Can you work these out from the model? Positions are in its coordinate system, mm. Face numbers are marked on the shaded views. A direction names the side the tool comes from. Give positions to 0.01 mm unless a question says otherwise; leave off trailing zeros. Order: outer loops, then holes, each group sorted by start corner. A loop starts at its lowest first (then second) coordinate and runs counter-clockwise, first axis right, second up.
```python
from build123d import *
from build123d.topology import SkipClean

# Parameters (mm, degrees)
BOSS_EXTRUDE1_START = -12.5
SKETCH1_W           = 27
SKETCH1_H           = 33
SKETCH1_R           = 7
BOSS_EXTRUDE1_DEPTH = 17
BOSS_EXTRUDE3_DEPTH = 12.5
BOSS_EXTRUDE4_START = 12.5
SKETCH1_5_R         = 5
BOSS_EXTRUDE4_DEPTH = 7
CHAMFER1_SIZE       = 5


with BuildPart() as part:
    # Sketch1 → Boss-Extrude1 (new body)
    with BuildSketch(Plane.XY.offset(BOSS_EXTRUDE1_START)):
        with Locations((-33.967633793, -25.34)):
            Rectangle(SKETCH1_W, SKETCH1_H)
        with Locations((-31.467633793, -22.84)):
            Circle(SKETCH1_R, mode=Mode.SUBTRACT)
    extrude(amount=BOSS_EXTRUDE1_DEPTH)

    # Sketch1<4> → Boss-Extrude3 (add, symmetric)
    with BuildSketch(Plane.XY):
        with BuildLine():
            ThreePointArc((28.205719919, -40.677666444), (11.699513519, -31.708687123), (1.506567213, -15.928912557))
            ThreePointArc((1.506567213, -15.928912557), (-3.134727468, -15.689916625), (-7.511545005, -14.127161486))
            Line((-7.511545005, -14.127161486), (-17.455249537, -8.84))
            Line((-17.455249537, -8.84), (-20.467633793, -8.84))
            Line((-20.467633793, -8.84), (-20.467633793, -41.84))
            Line((-20.467633793, -41.84), (-18.535800645, -41.84))
            ThreePointArc((-18.535800645, -41.84), (-12.817002571, -43.63662578), (-9.153112508, -48.38093028))
            ThreePointArc((-9.153112508, -48.38093028), (-5.868981967, -55.429445297), (-1.467633793, -61.84))
            Line((-1.467633793, -61.84), (11.532366207, -61.84))
            Line((11.532366207, -61.84), (28.205719919, -40.677666444))
        make_face()
    extrude(amount=BOSS_EXTRUDE3_DEPTH, both=True)

    # Sketch1<5> → Boss-Extrude4 (add)
    with BuildSketch(Plane.XY.offset(BOSS_EXTRUDE4_START)):
        with BuildLine():
            Line((37.532366207, -3.84), (15.532366207, -3.84))
            ThreePointArc((15.532366207, -3.84), (10.445897028, -12.1195394), (1.506567213, -15.928912557))
            ThreePointArc((1.506567213, -15.928912557), (11.699513519, -31.708687123), (28.205719919, -40.677666444))
            Line((28.205719919, -40.677666444), (37.532366207, -28.84))
            Line((37.532366207, -28.84), (37.532366207, -3.84))
        make_face()
        with Locations((25.532366207, -18.84)):
            Circle(SKETCH1_5_R, mode=Mode.SUBTRACT)
    boss_extrude4 = extrude(amount=-BOSS_EXTRUDE4_DEPTH)

    # Mirror1: Boss-Extrude4 across plane
    with SkipClean():  # the faces are left unmerged after this step: merging them gives an invalid solid
        add(boss_extrude4.mirror(Plane.XY))

    # Chamfer1
    chamfer1_edges = [part.edges().sort_by_distance(p)[0] for p in [
        (-47.467633793, -41.84, -4),
        (-47.467633793, -8.84, -4),
        (37.532366207, -3.84, 9),
        (37.532366207, -3.84, -9),
    ]]
    chamfer(chamfer1_edges, length=CHAMFER1_SIZE)


solid = part.part
```
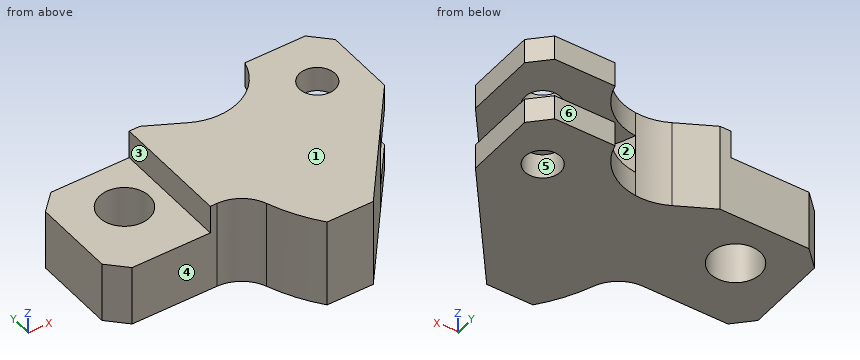
1) We'd pull the mould along Y, two halves only. Please class the marked faces 4, 5 and 6: +Y half, -Y half, draft (parallel to the pull), parting line (faces both ways), or undercut.
2) If I drill on line 1 (Z direction, x = 15.5, y = -30); line 2 (Y direction, x = -23.5, z = -8.25); line 3 (Y direction, x = 22, z = -6), over which ranges is the centre line in solid material (lowest first)?
3) I'm going to push flat-ended pins straight in: pin 1 Ø2.5 at (y, z) = (-23.5, 6.5) entering from -X; pin 2 Ø6 at (y, z) = (-35.5, 3) entering from +X; pin 3 Ø12 at (x, z) = (21.5, 1) entering from -Y. Where does each tip first touch, or does it pass through?
4) Suppose I cut it at B-B (z = 0). Please give me the cut outline in (x, y).
5) Suppose I cut it at C-C (y = -18.84). Please give me the cut outline in (x, z).
6) Suppose I cut it at A-A (z = -11). Please give me the cut outline in (x, y).
7) Suppose I cut it at D-D (x = 12.5). Please give me the cut outline in (y, z), and give its area (3 significant figures).
8) Which directions (+Z, -Z, +X, -X, +Y, -Y) give clear straight access to the entire face, cutting with the end or side of a thin tool? Please do the marked faces 1, 2 and 3.
Results:
1. face 4: -Y half
1. face 5: undercut
1. face 6: +Y half
2. line 1: z = -12.5 to -5.5, 5.5 to 12.5
2. line 2: y = -41.84 to -8.84
2. line 3: y = -48.55 to -22.38, -15.3 to -3.84
3. pin 1: stops at x = -20.47
3. pin 2: stops at x = 33.59
3. pin 3: stops at y = -56.8
4. outline: (-47.47, -36.84) - (-42.47, -41.84) - (-18.54, -41.84) arc R10 cw to (-9.15, -48.38) arc R47 ccw to (-1.47, -61.84) - (11.53, -61.84) - (28.21, -40.68) arc R38 cw to (1.51, -15.93) arc R16 cw to (-7.51, -14.13) - (-17.46, -8.84) - (-42.47, -8.84) - (-47.47, -13.84) - close; hole circle Ø14 at (-31.47, -22.84)
5. outline: (-47.47, -12.5) - (-37.21, -12.5) - (-37.21, 4.5) - (-47.47, 4.5) - close; (-25.72, -12.5) - (20.53, -12.5) - (20.53, -5.5) - (2.62, -5.5) - (2.62, 5.5) - (20.53, 5.5) - (20.53, 12.5) - (-20.47, 12.5) - (-20.47, 4.5) - (-25.72, 4.5) - close; (30.53, -12.5) - (37.53, -12.5) - (37.53, -5.5) - (30.53, -5.5) - close; (30.53, 5.5) - (37.53, 5.5) - (37.53, 12.5) - (30.53, 12.5) - close
6. outline: (-47.47, -36.84) - (-42.47, -41.84) - (-18.54, -41.84) arc R10 cw to (-9.15, -48.38) arc R47 ccw to (-1.47, -61.84) - (11.53, -61.84) - (37.53, -28.84) - (37.53, -8.84) - (32.53, -3.84) - (15.53, -3.84) arc R16 cw to (-7.51, -14.13) - (-17.46, -8.84) - (-42.47, -8.84) - (-47.47, -13.84) - close; hole circle Ø14 at (-31.47, -22.84); hole circle Ø10 at (25.53, -18.84)
7. outline: (-60.61, -12.5) - (-9.99, -12.5) - (-9.99, -5.5) - (-32.43, -5.5) - (-32.43, 5.5) - (-9.99, 5.5) - (-9.99, 12.5) - (-60.61, 12.5) - close
7. area: 1,020 mm2
8. face 1: +Z, +X, -X, +Y, -Y
8. face 2: +X, +Y
8. face 3: +Z, -X, +Y, -Y
